Geometry: final body of the model. Coordinates: model frame, mm. A direction names the side the tool comes from. Give positions to 0.01 mm unless a question says otherwise; leave off trailing zeros. Loops run counter-clockwise (first coordinate to the right, second up) from the corner with the lowest first, then second, coordinate; pieces in that order, holes last. Notation, with made-up numbers: (-0.75, -18) - (45.25, -18) arc R6 ccw to (45.25, -13) - close; hole circle Ø3 at (83, 37). An arc over 180 degrees is marked (long way). Answer in a Markdown table with one row per item.
from build123d import *

# Parameters (mm, degrees)
F1_DEPTH = 50


with BuildPart() as f1:
    # F0 (on Front) → F1 (new body)
    with BuildSketch(Plane.XZ):
        Polygon((-54.376826, 94.42836), (-54.376826, 103.330544), (-74.380621, 103.330544), (-74.380621, 39.594981), (-77.379836, 34.080958), (-73.407053, 31.455231), (-73.407053, -2.616242), (2.095642, -2.616242), (2.095642, 44.139318), (-24.235287, 44.139318), (-35.565158, 61.786109), (-34.995204, 68.73957), (-48.275114, 77.498662), align=None)
        Polygon((-63.30613, 51.583886), (-70.380621, 63.319154), (-70.380621, 99.330544), (-58.376826, 99.330544), (-58.376826, 85.526176), (-55.210922, 81.59513), (-54.556411, 76.849923), (-39.175387, 66.704988), (-39.993525, 56.723688), (-42.759668, 53.943455), (-39.323483, 49.361873), (-34.610999, 52.896235), (-22.848731, 34.575965), (-8.449475, 36.048617), (-5.667799, 40.139318), (-1.904358, 35.394106), (-1.904358, 1.383758), (-69.407053, 1.383758), (-69.407053, 25.991378), (-67.709148, 31.495143), (-72.112158, 35.394106), align=None, mode=Mode.SUBTRACT)
    extrude(amount=F1_DEPTH)


solid = f1.part
Q1. Cut plane B-B (z = 5). Output: boundary loops of the cut face in (x, y), and give its area (3 significant figures).
Check values:
| item | result |
|---|---|
| outline | (-73.41, -50) - (-69.41, -50) - (-69.41, 0) - (-73.41, 0) - close; (-1.9, -50) - (2.1, -50) - (2.1, 0) - (-1.9, 0) - close |
| area | 400 mm² |
Q2. Reachability of faces 1 (the flat face through (-35.284, -24.65, 65.214)), 2 (the flat face through (-69.88, -24.65, 33.42)), 3 (the flat face through (-73.407, -25, 15)), 4 (the flat face through (-54.377, -25, 99)) from +Z, -Z, +X, -X, +Y, -Y: full face, straight path, thin tool, end or side. Return the list, or none.
Check values:
| item | result |
|---|---|
| face 1 | +X, +Y, -Y |
| face 2 | +Y, -Y |
| face 3 | -Z, -X, +Y, -Y |
| face 4 | +Z, +X, +Y, -Y |
Q3. Cut plane C-C (x = -28). Output: boundary loops of the cut face in (y, z), and give its area (3 significant figures).
Check values:
| item | result |
|---|---|
| outline | (-50, -2.62) - (0, -2.62) - (0, 1.38) - (-50, 1.38) - close; (-50, 42.6) - (0, 42.6) - (0, 50) - (-50, 50) - close |
| area | 570 mm² |
Q4. First-contact query: pin 1 (10 mm diameter, centred on y = -27, z = 83, fed in from +X); pin 2 (4 mm diameter, centred on y = -27, z = 20.5, fed in from -X); pin 3 (8 mm diameter, centred on x = -68.5, z = 81, fed in from -Y); pin 4 (2.5 mm diameter, centred on y = -26, z = 97, fed in from +X). Flat tips, straight axial feed; report the tip coordinate or a pass-through.
Check values:
| item | result |
|---|---|
| pin 1 | x = -48.46 |
| pin 2 | x = -73.41 |
| pin 3 | y = -50 |
| pin 4 | x = -54.38 |
Q5. Draft query along Z for faces 5 (the flat face through (-64, -25, 99.331)), 6 (the flat face through (-64, -25, 103.331)), 7 (the flat face through (-41.066, -24.65, 51.685)), 8 (the flat face through (-38, -50, 55)). Return one class per face: pulls with the +Z half, pulls with the -Z half, needs draft (parallel to the pull), parting line crosses it, or undercut.
Check values:
| item | result |
|---|---|
| face 5 | undercut |
| face 6 | pulls with the +Z half |
| face 7 | undercut |
| face 8 | needs draft |
Q6. Material intervals for line 1 along X through (y, z) = (-43, 15.5); line 2 along Z through (x, y) = (-66.5, -33); line 3 along Z through (x, y) = (-67, -14), sorted ascending.
Check values:
| item | result |
|---|---|
| line 1 | -73.41 to -69.41, -1.9 to 2.1 |
| line 2 | -2.62 to 1.38, 45.71 to 56.88, 99.33 to 103.33 |
| line 3 | -2.62 to 1.38, 44.79 to 57.71, 99.33 to 103.33 |
